from build123d import *

# Parameters (mm, degrees)
EXTRUDE_1_DEPTH      = 100
EXTRUDE_1_DEPTH_BACK = 150
SKETCH_2_R           = 8.5
CUT_EXTRUDE_1_DEPTH  = 173.336879396


with BuildPart() as part:
    # Эскиз1 → Бобышка-Вытянуть1 (new, two sides: drawn at the far end of the back side and taken through both)
    with BuildSketch(Plane(origin=(0, 0, 0), x_dir=(1, 0, 0), z_dir=(0, 1, 0)).offset(-EXTRUDE_1_DEPTH_BACK)):
        with BuildLine():
            Line((-56, 0), (-4, 0))
            ThreePointArc((-4, 0), (-1.171572875, -1.171572875), (0, -4))
            Line((0, -4), (0, -56))
            ThreePointArc((0, -56), (-1.171572875, -58.828427125), (-4, -60))
            Line((-4, -60), (-56, -60))
            ThreePointArc((-56, -60), (-58.828427125, -58.828427125), (-60, -56))
            Line((-60, -56), (-60, -4))
            ThreePointArc((-60, -4), (-58.828427125, -1.171572875), (-56, 0))
        make_face()
        with BuildLine():
            Line((-53, -4), (-7, -4))
            ThreePointArc((-7, -4), (-4.878679656, -4.878679656), (-4, -7))
            Line((-4, -7), (-4, -53))
            ThreePointArc((-4, -53), (-4.878679656, -55.121320344), (-7, -56))
            Line((-7, -56), (-53, -56))
            ThreePointArc((-53, -56), (-55.121320344, -55.121320344), (-56, -53))
            Line((-56, -53), (-56, -7))
            ThreePointArc((-56, -7), (-55.121320344, -4.878679656), (-53, -4))
        make_face(mode=Mode.SUBTRACT)
    extrude(amount=EXTRUDE_1_DEPTH + EXTRUDE_1_DEPTH_BACK)

    # Эскиз2 → Вырез-Вытянуть1 (cut, through all)
    with BuildSketch(Plane.XY.offset(60)):
        with Locations((-30, 50)):
            Circle(SKETCH_2_R)
    extrude(amount=-CUT_EXTRUDE_1_DEPTH, mode=Mode.SUBTRACT)


solid = part.part
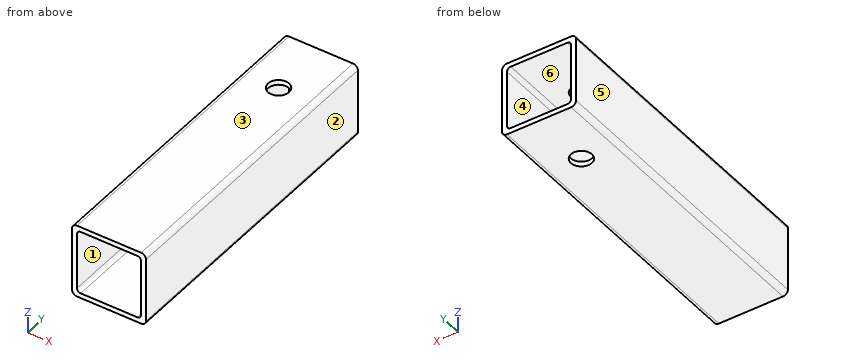
Could you check a few things on this model? Use its own coordinates, in mm. Face numbers are marked on the shaded views. A direction names the side the tool comes from. Give positions to 0.01 mm unless a question says otherwise; leave off trailing zeros. Order: outer loops, then holes, each group sorted by start corner. A loop starts at its lowest first (then second) coordinate and runs counter-clockwise, first axis right, second up. Notation, with made-up numbers: (17, -26.5) -> (46, -26.5) arc R25 ccw to (46, 2.5) -> close; hole circle Ø9 at (62, -19.75). An arc over 180 degrees is marked (long way). Return JSON: item names as keys, results as strings.
1. Imagine slicing it at B-B on y = 50. List the corners of the cut face in (x, z) for me, then the cut area to 3 significant figures.
Answer list:
{"outline": "(-60, 4) arc R4 ccw to (-56, 0) -> (-38.5, 0) -> (-38.5, 4) -> (-53, 4) arc R3 cw to (-56, 7) -> (-56, 53) arc R3 cw to (-53, 56) -> (-38.5, 56) -> (-38.5, 60) -> (-56, 60) arc R4 ccw to (-60, 56) -> close; (-21.5, 0) -> (-4, 0) arc R4 ccw to (0, 4) -> (0, 56) arc R4 ccw to (-4, 60) -> (-21.5, 60) -> (-21.5, 56) -> (-7, 56) arc R3 cw to (-4, 53) -> (-4, 7) arc R3 cw to (-7, 4) -> (-21.5, 4) -> close", "area": "754 mm2"}
2. Imagine slicing it at A-A on x = -11. List the corners of the cut face in (y, z) for me, then the cut area to 3 significant figures.
Answer list:
{"outline": "(-150, 0) -> (100, 0) -> (100, 4) -> (-150, 4) -> close; (-150, 56) -> (100, 56) -> (100, 60) -> (-150, 60) -> close", "area": "2,000 mm2"}
3. On a 3-axis mill with a long thin cutter (end or side, diameter ignored), from which of +Z, -Z, +X, -X, +Y, -Y can I reach the whole of each face in a straight line? I mean the marked faces 1 and 2. Say none if no direction works.
Answer list:
{"face 1": "+Y, -Y", "face 2": "+Z, -Z, +X, +Y, -Y"}
4. Imagine slicing it at D-D on z = 42.5. List the corners of the cut face in (x, y) for me.
Answer list:
{"outline": "(-60, -150) -> (-56, -150) -> (-56, 100) -> (-60, 100) -> close; (-4, -150) -> (0, -150) -> (0, 100) -> (-4, 100) -> close"}
5. Imagine slicing it at C-C on x = -30. List the corners of the cut face in (y, z) for me.
Answer list:
{"outline": "(-150, 0) -> (41.5, 0) -> (41.5, 4) -> (-150, 4) -> close; (-150, 56) -> (41.5, 56) -> (41.5, 60) -> (-150, 60) -> close; (58.5, 0) -> (100, 0) -> (100, 4) -> (58.5, 4) -> close; (58.5, 56) -> (100, 56) -> (100, 60) -> (58.5, 60) -> close"}
6. I need wall thicknesses on line 1 (Z direction, x = -21.5, y = -86); line 2 (Y direction, x = -30, z = 1.6); line 3 (X direction, y = -54, z = 8). Which ranges of each line are inside material? Lowest first, please. Write a range as from..to.
Answer list:
{"line 1": "z = 0..4, 56..60", "line 2": "y = -150..41.5, 58.5..100", "line 3": "x = -60..-56, -4..0"}
7. Thinking about a two-plate mould opening in Z: for the marked faces 3, 4, 5 and 6, which applies, pulls with the +Z half, pulls with the -Z half, needs draft (parallel to the pull), parting line crosses it, or undercut?
Answer list:
{"face 3": "pulls with the +Z half", "face 4": "undercut", "face 5": "needs draft", "face 6": "undercut"}
